from build123d import *

# Parameters (mm, degrees)
F1_DEPTH = 523.24
F2_R     = 4.572
F4_D     = 8.1
F4_DEPTH = 20
F6_D     = 8
F6_DEPTH = 10


with BuildPart() as f1:
    # F0 (on Front) → F1 (new body)
    with BuildSketch(Plane.XZ):
        Polygon((0, 101.6), (0, 0), (50.8, 0), (50.8, 5.842), (3.81, 5.842), (3.81, 95.758), (50.8, 95.758), (50.8, 101.6), align=None)
    extrude(amount=-F1_DEPTH)

    # F2
    f2_edges = [f1.edges().sort_by_distance(p)[0] for p in [
        (3.81, 261.62, 5.842),
        (3.81, 261.62, 95.758),
    ]]
    fillet(f2_edges, radius=F2_R)

    # F4
    with Locations(Plane.XY.offset(101.6)):
        with Locations((17.4625, 503.24), (17.4625, 20)):
            Hole(F4_D / 2, depth=F4_DEPTH)

    # F6
    with Locations(Plane(origin=(0, 0, 0), x_dir=(1, 0, 0), z_dir=(0, 0, -1))):
        with Locations((25, -19), (25, -504.24)):
            Hole(F6_D / 2, depth=F6_DEPTH)


solid = f1.part
The listing builds one solid part. Answer for the finished solid, in the listing's coordinates (mm). A direction names the side the tool comes from. Coordinates: 2 decimals unless noted, no trailing zeros. Write each loop counter-clockwise with the first axis right and the second up, starting at its lowest first coordinate (ties: lowest second). Pieces come first, ordered by that corner, then holes. Notation, with made-up numbers: (-10, -26) -> (37, -26) arc R17 ccw to (37, 3) -> close; hole circle Ø5 at (65.5, -3). An arc over 180 degrees is marked (long way). One line per question, with ' | ' between items.
1. Straight lines are drawn through the part: line 1 (Y direction, x = 25, z = 2.55); line 2 (X direction, y = 503, z = 98); line 3 (Z direction, x = 24, y = 360). For each, find the intervals that lie inside material, in ascending order.
Verdict:
line 1: y = 0 to 15, 23 to 500.24, 508.24 to 523.24 | line 2: x = 0 to 13.42, 21.51 to 50.8 | line 3: z = 0 to 5.84, 95.76 to 101.6
2. Section B-B (y = 274.5) is taken. Determine the outline of the cut face in (x, z), and give its area (3 significant figures).
Verdict:
outline: (0, 0) -> (50.8, 0) -> (50.8, 5.84) -> (8.38, 5.84) arc R4.57 cw to (3.81, 10.41) -> (3.81, 91.19) arc R4.57 cw to (8.38, 95.76) -> (50.8, 95.76) -> (50.8, 101.6) -> (0, 101.6) -> close | area: 945 mm^2
3. Section C-C (z = 30) is taken. Determine the outline of the cut face in (x, y), and give its area (3 significant figures).
Verdict:
outline: (0, 0) -> (3.81, 0) -> (3.81, 523.24) -> (0, 523.24) -> close | area: 1,990 mm^2
4. For a pull along X with two mould halves and no side action, classify faces 1 (the cylindrical face through (18.34, 499.286, 98.638)), 2 (the flat face through (3.81, 258, 50)), 3 (the cylindrical face through (13.72, 18.45, 98.64)), 4 (the flat face through (3, 0, 59)) as released by +X, released by -X, zero draft, split by the parting line, or undercut.
Verdict:
face 1: undercut | face 2: released by +X | face 3: undercut | face 4: zero draft
5. Section A-A (x = 43) is taken. Determine the outline of the cut face in (y, z).
Verdict:
outline: (0, 0) -> (523.24, 0) -> (523.24, 5.84) -> (0, 5.84) -> close; (0, 95.76) -> (523.24, 95.76) -> (523.24, 101.6) -> (0, 101.6) -> close
6. Which of the six approach directions +Z, -Z, +X, -X, +Y, -Y give full straight-line access (tool end or side, diameter ignored) to faces 5 (the flat face through (30, 258, 5.842)), 6 (the flat face through (3, 523.24, 59))?
Verdict:
face 5: +X, +Y, -Y | face 6: +Z, -Z, +X, -X, +Y
7. Given pin 1 Ø4 at (x, y) = (45.5, 214) entering from -Z; pin 2 Ø5 at (y, z) = (281.5, 49) entering from +X; pin 3 Ø6.5 at (x, y) = (25, 19) entering from -Z, each flat-ended and moving along its own axis, determine where each tip first touches the part or whether it passes through.
Verdict:
pin 1: stops at z = 0 | pin 2: stops at x = 3.81 | pin 3: stops at z = 95.76
